from build123d import *

# Parameters (mm, degrees)
SKETCH2_R           = 16
BOSS_EXTRUDE1_DEPTH = 40
SKETCH3_R           = 3.75
CUT_EXTRUDE1_DEPTH  = 8.5
BOSS_EXTRUDE3_DEPTH = 40


with BuildPart() as part:
    # Sketch2 → Boss-Extrude1 (new body)
    with BuildSketch(Plane(origin=(0, 0, 0), x_dir=(0, 0, -1), z_dir=(1, 0, 0))):
        Circle(SKETCH2_R)
    extrude(amount=BOSS_EXTRUDE1_DEPTH)

    # Sketch3 → Cut-Extrude1 (cut)
    with BuildSketch(Plane(origin=(0, 0, 0), x_dir=(0, 0, -1), z_dir=(1, 0, 0))):
        Circle(SKETCH3_R)
    extrude(amount=CUT_EXTRUDE1_DEPTH, mode=Mode.SUBTRACT)

    # Sketch4 → Boss-Extrude3 (add, through all)
    with BuildSketch(Plane(origin=(0, 0, 0), x_dir=(0, 0, -1), z_dir=(1, 0, 0))):
        Polygon((10, 12.489995997), (-10, 12.489995997), (-10, 15.822191594), (-10, 22.739406358), (10, 22.739406358), align=None)
    extrude(amount=BOSS_EXTRUDE3_DEPTH)


solid = part.part
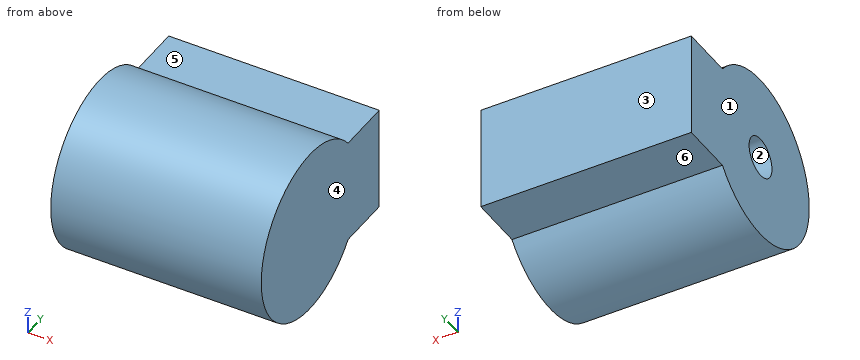
The model under review builds one solid part; all positions refer to its coordinate system, in mm. Face numbers are marked on the shaded views. A direction names the side the tool comes from. Round coordinates to 2 decimals unless told otherwise and drop trailing zeros. Loops run counter-clockwise (first coordinate to the right, second up) from the corner with the lowest first, then second, coordinate; pieces in that order, holes last. Notation, with made-up numbers: (87, -11) -> (107, -11) arc R18 ccw to (107, 16) -> close; hole circle Ø11 at (24.25, 53). An arc over 180 degrees is marked (long way). Answer as CSV lines item,"result".
1) Add section D-D on x = 33.5. Write out the cut boundary in (y, z), plus the area to 3 significant figures.
Geometry results:
outline,"(12.49, -10) -> (22.74, -10) -> (22.74, 10) -> (12.49, 10) arc R16 ccw (long way) to start"
area,"961 mm²"
2) Tool access review of the marked faces 4, 5 and 6: name each direction out of +Z, -Z, +X, -X, +Y, -Y from which nothing blocks a thin tool from reaching the whole face with its end or side.
Geometry results:
face 4,"+Z, -Z, +X, +Y, -Y"
face 5,"+Z, +X, -X, +Y"
face 6,"-Z, +X, -X, +Y"
3) To check wall thickness, follow line 1 along Y through (x, z) = (3.5, 0); line 2 along Z through (x, y) = (32, 18.5); line 3 along Z through (x, y) = (38.5, -6). State the ranges of each line that lie inside material, in increasing order. Write a range as from..to.
Geometry results:
line 1,"y = -16..-3.75, 3.75..22.74"
line 2,"z = -10..10"
line 3,"z = -14.83..14.83"
4) For P1, Ø12, axis at x = 20.5, z = -9.5, coming from the -Y side; P2, Ø4, axis at x = 16, z = 8.5, coming from the -Y side; P3, Ø11.5, axis at x = 14, y = 17.5, coming from the +Z side; P4, Ø1, axis at y = 13.5, z = 11.5, coming from the -X side, all flat-tipped, find the tip position at first contact; note any pin that passes through.
Geometry results:
P1,"stops at y = -15.61"
P2,"stops at y = -14.62"
P3,"stops at z = 10.86"
P4,"passes through"
5) Add section A-A on x = 7. Write out the cut boundary in (y, z), plus the area to 3 significant figures.
Geometry results:
outline,"(12.49, -10) -> (22.74, -10) -> (22.74, 10) -> (12.49, 10) arc R16 ccw (long way) to start; hole circle Ø7.5 at (0, 0)"
area,"917 mm²"
6) Add section C-C on z = 0. Write out the cut boundary in (x, y).
Geometry results:
outline,"(0, -16) -> (40, -16) -> (40, 22.74) -> (0, 22.74) -> (0, 3.75) -> (8.5, 3.75) -> (8.5, -3.75) -> (0, -3.75) -> close"
7) Draft analysis for pull direction Y (two halves, no side actions). For the marked faces 1, 2 and 3, state which applies: pulls with the +Y half, pulls with the -Y half, needs draft (parallel to the pull), parting line crosses it, or undercut.
Geometry results:
face 1,"needs draft"
face 2,"undercut"
face 3,"pulls with the +Y half"
8) Add section B-B on y = 0. Write out the cut boundary in (x, z), plus the area to 3 significant figures.
Geometry results:
outline,"(0, -16) -> (40, -16) -> (40, 16) -> (0, 16) -> (0, 3.75) -> (8.5, 3.75) -> (8.5, -3.75) -> (0, -3.75) -> close"
area,"1,220 mm²"
